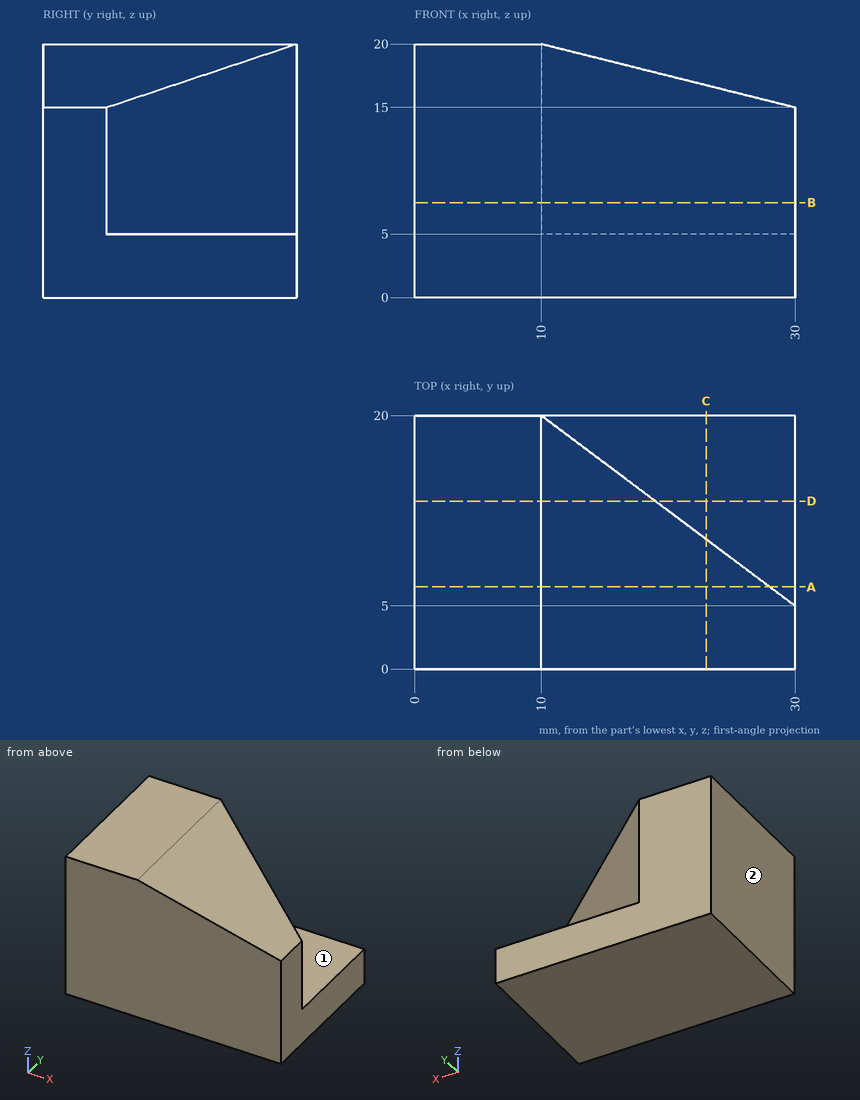
Verification items for this drawing (mm, ordinates from the low corner). A direction names the side the tool comes from. Give positions to 0.01 mm unless a question says otherwise; leave off trailing zeros. Loops run counter-clockwise (first coordinate to the right, second up) from the corner with the lowest first, then second, coordinate; pieces in that order, holes last. Notation, with made-up numbers: M 71.5,81 L 98.5,81 A34 cw 98.5,120 Z; hole C 72,81.25 d4. An arc over 180 degrees is marked long. Answer in a Markdown table with one row per item.
1) Cross-section at C-C (x = 23). Enter the section's corners in (y, z), plus the area to 3 significant figures.
Solutions:
| item | result |
|---|---|
| outline | M 0,0 L 20,0 L 20,5 L 10.25,5 L 10.25,16.75 L 0,16.75 Z |
| area | 220 mm^2 |
2) Thickness scan on line 1 (Z direction, x = 18, y = 15.5); line 2 (Y direction, x = 26.5, z = 14) (3 decimals); line 3 (X direction, y = 14.75, z = 9.5). Record the ranges inside material, lowest first.
Solutions:
| item | result |
|---|---|
| line 1 | z = 0 to 5 |
| line 2 | y = 0 to 7.625 |
| line 3 | x = 0 to 17 |
3) Tool access check on the marked faces 1 and 2. Record the directions out of +Z, -Z, +X, -X, +Y, -Y that give a thin tool (end or side, any length) a straight path to the whole face; none if there is none.
Solutions:
| item | result |
|---|---|
| face 1 | +Z, +X, +Y |
| face 2 | +Z, -Z, -X, +Y, -Y |
4) Cross-section at B-B (z = 7.5). Enter the section's corners in (x, y).
Solutions:
| item | result |
|---|---|
| outline | M 0,0 L 30,0 L 30,5 L 10,20 L 0,20 Z |
5) Cross-section at A-A (y = 6.5). Enter the section's corners in (x, z).
Solutions:
| item | result |
|---|---|
| outline | M 0,0 L 30,0 L 30,5 L 28,5 L 28,15.5 L 10,20 L 0,20 Z |
6) Cross-section at D-D (y = 13.25). Enter the section's corners in (x, z).
Solutions:
| item | result |
|---|---|
| outline | M 0,0 L 30,0 L 30,5 L 19,5 L 19,17.75 L 10,20 L 0,20 Z |
7) Depth check by flat-ended pin: pin 1 (4 mm diameter, centred on y = 12.5, z = 17, fed in from +X); pin 2 (4.5 mm diameter, centred on x = 24.5, y = 15, fed in from +Z); pin 3 (1.5 mm diameter, centred on x = 15, z = 16, fed in from +Y). Enter the tip coordinate at first touch or a pass-through.
Solutions:
| item | result |
|---|---|
| pin 1 | stops at x = 22.66 |
| pin 2 | stops at z = 5 |
| pin 3 | stops at y = 16.81 |
